Work out the finished part from the listing and answer in its coordinate system (mm). A direction names the side the tool comes from. Give positions to 0.01 mm unless a question says otherwise; leave off trailing zeros. Order: outer loops, then holes, each group sorted by start corner. A loop starts at its lowest first (then second) coordinate and runs counter-clockwise, first axis right, second up.
Autodesk Inventor part; units mm, degrees
ref_plane "YZ Plane" through (0, 0, 0) normal (1, 0, 0) x (0, 1, 0)
ref_plane "XZ Plane" through (0, 0, 0) normal (0, 1, 0) x (-1, 0, 0)
ref_plane "XY Plane" through (0, 0, 0) normal (0, 0, 1) x (1, 0, 0)
sketch "Эскиз1" plane through (0, 0, 0) normal (0, 1, 0) x (-1, 0, 0)
  line L0 (0, 0) -> (47.5295, 0)
  line L1 (0, 0) -> (-53.4705, 0)
  line L2 (47.5295, 0) -> (-53.4705, 0)
  line L3 (-53.4705, 0) -> (-53.4705, 10)
  line L4 (-53.4705, 10) -> (47.5295, 10)
  line L5 (47.5295, 10) -> (47.5295, 0)
  dimension "d0" = 101
  dimension "d1" = 10
extrude "Выдавливание1" add sketch "Эскиз1" along normal blind 4
sketch "Эскиз2" plane through (-47.5295, 0, 10) normal (0, 0, 1) x (1, 0, 0)
  line L0 (0, 4) -> (101, 4)
  line L1 (0, 4) -> (50.5, 4)
  line L2 (30.5, 0) -> (70.5, 0)
  line L3 (70.5, 0) -> (70.5, 4)
  line L4 (70.5, 4) -> (30.5, 4)
  line L5 (30.5, 4) -> (30.5, 0)
  line L6 (30.5, 0) -> (70.5, 4) construction
  line L7 (70.5, 0) -> (30.5, 4) construction
  point P0 (47.5295, 0)
  point P1 (50.5, 2)
  point P2 (30.5, 2)
  point P3 (70.5, 2)
  dimension "d4" = 50.5
  dimension "d5" = 40
  dimension "d6" = 4
extrude "Выдавливание2" add sketch "Эскиз2" along normal blind 20
sketch "Эскиз3" plane through (0, 4, 0) normal (0, 1, 0) x (1, 0, 0)
  line L0 (-17.0295, -30) -> (22.9705, -30)
  line L1 (22.9705, -10) -> (22.9705, -30)
  line L2 (-17.0295, -30) -> (22.9705, -30)
  line L3 (22.9705, -30) -> (22.9705, -26)
  line L4 (22.9705, -26) -> (-17.0295, -26)
  line L5 (-17.0295, -26) -> (-17.0295, -30)
  point P0 (0, 0)
  dimension "d9" = 4
extrude "Выдавливание3" add sketch "Эскиз3" along normal blind 10
sketch "Эскиз4" plane through (53.4705, 0, 10) normal (1, 0, 0) x (0, 0, -1)
  line L0 (0, 4) -> (10, 4)
  line L1 (0, 4) -> (27, 4)
  line L2 (27, 4) -> (27, 0)
  line L3 (27, 0) -> (0, 0)
  line L4 (0, 0) -> (0, 4)
  line L5 (10, 0) -> (10, 4)
  dimension "d12" = 17
extrude "Выдавливание4" add sketch "Эскиз4" along normal blind 4
sketch "Эскиз5" plane through (-47.5295, 0, 0) normal (-1, 0, 0) x (0, 0, 1)
  line L0 (-17, 4) -> (0, 4)
  line L1 (10, 0) -> (-17, 0)
  line L2 (-17, 0) -> (-17, 4)
  line L3 (-17, 4) -> (10, 4)
  line L4 (10, 4) -> (10, 0)
  point P0 (0, 0)
  point P1 (0, 4)
extrude "Выдавливание5" add sketch "Эскиз5" along normal blind 4
sketch "Эскиз6" plane through (-47.5295, 0, 0) normal (1, 0, 0) x (0, 0, -1)
  circle A0 centre (14.9, 2.0073) radius 1.5
  line L0 (14.9, 2.0073) -> (17, 2)
  line L1 (17, 4) -> (17, 0)
  point P0 (0, 0)
  dimension "d17" = 3
  dimension "d18" = 2.1
extrude "Выдавливание6" add sketch "Эскиз6" along normal blind 4
sketch "Эскиз7" plane through (53.4705, 0, 10) normal (-1, 0, 0) x (0, 0, 1)
  circle A0 centre (-24.9, 2.0073) radius 1.5
  circle A1 centre (-24.9, 2.0073) radius 1.5
  point P0 (-10, 0)
extrude "Выдавливание7" add sketch "Эскиз7" along normal blind 4
properties part number "крюк"
1. The mould has two halves that part along X. Classify faces 5 (the face through (-50, 2, -17)), 6 (the face through (22.97, 3.8, 22.1)), 7 (the face through (-51.53, 2, -4)), 8 (the face through (-45.56, 1.94, -13.4)): pulls with the +X half, pulls with the -X half, needs draft (parallel to the pull), parting line crosses it, or undercut.
Findings below:
face 5: needs draft
face 6: pulls with the +X half
face 7: pulls with the -X half
face 8: undercut
2. Given P1, Ø1.2, axis at x = -36.5, y = 1, coming from the +Z side; P2, Ø13, axis at x = -3, z = 0, coming from the +Y side; P3, Ø8, axis at x = 10.5, y = 9, coming from the -Z side; P4, Ø2, axis at x = 0, z = 15, coming from the -Y side, each flat-ended and moving along its own axis, determine where each tip first touches the part or whether it passes through.
Findings below:
P1: stops at z = 10
P2: stops at y = 4
P3: stops at z = 26
P4: stops at y = 0
3. The part is cut by section D-D (y = 11). Write down the section's boundary in (x, z).
Findings below:
outline: (-17.03, 26) - (22.97, 26) - (22.97, 30) - (-17.03, 30) - close
4. The part is cut by section C-C (z = 14.5). Write down the section's boundary in (x, y), then the cut area to 3 significant figures.
Findings below:
outline: (-17.03, 0) - (22.97, 0) - (22.97, 4) - (-17.03, 4) - close
area: 160 mm2
5. The part is cut by section A-A (z = -11). Write down the section's boundary in (x, y), then the cut area to 3 significant figures.
Findings below:
outline: (-51.53, 0) - (-47.53, 0) - (-47.53, 4) - (-51.53, 4) - close; (53.47, 0) - (57.47, 0) - (57.47, 4) - (53.47, 4) - close
area: 32.0 mm2
6. The part is cut by section B-B (x = 7.5). Write down the section's boundary in (y, z), then the cut area to 3 significant figures.
Findings below:
outline: (0, 0) - (4, 0) - (4, 26) - (14, 26) - (14, 30) - (0, 30) - close
area: 160 mm2
7. Which of the six approach directions +Z, -Z, +X, -X, +Y, -Y give full straight-line access (tool end or side, diameter ignored) to faces 1 (the face through (-34, 2, 10)), 2 (the face through (49.47, 2, -15)), 3 (the face through (3, 4, 8)), 4 (the face through (51.5, 1.94, -16.4))?
Findings below:
face 1: +Z, -X, +Y, -Y
face 2: -Z, +Y, -Y
face 3: -Z, +X, -X, +Y
face 4: none
8. Straight lines are drawn through the part: probe 1 along X at (y, z) = (0.5, -6); probe 2 along Z at (x, y) = (7, 9); probe 3 along Z at (x, y) = (6, 3.5). For each, find the intervals that lie inside material, in ascending order.
Findings below:
probe 1: x = -51.53 to -47.53, 53.47 to 57.47
probe 2: z = 26 to 30
probe 3: z = 0 to 30
